Could you check a few things on this model? Use its own coordinates, in mm. A direction names the side the tool comes from. Coordinates: 2 decimals unless noted, no trailing zeros. Loops run counter-clockwise (first coordinate to the right, second up) from the corner with the lowest first, then second, coordinate; pieces in that order, holes last. Notation, with made-up numbers: (36.5, 84) - (48.5, 84) arc R28 cw to (48.5, 122) - close; hole circle Ø11 at (86, 30). An arc over 180 degrees is marked (long way). One line per item, written item: value. Start each with the question number.
(1) If we section it at B-B on y = 10.5: Write out the boundary of the cut face in (x, z).
(2) If we section it at D-D on y = 6.5: Write out the boundary of the cut face in (x, z), then the cut area to 3 significant figures.
(3) I'm going to push flat-ended pins straight in: P1, Ø10, axis at x = -13, z = -23, coming from the +Y side; P2, Ø2, axis at x = -11.5, z = -1.5, coming from the +Y side; P3, Ø0.6, axis at y = 16, z = -2, coming from the -X side. Where does each tip first touch, or does it pass through?
(4) If I drill on line 1 along X through (y, z) = (14, -10); line 2 along X through (y, z) = (1.5, -10.5); line 3 along Z through (x, y) = (-6, 6.25), over which ranges is the centre line in solid material (lowest first)? Write a range as from..to.
(5) If we mould it in two halves opening along Y, with no side actions, what happens to faces 1 (the face through (-2.54, 9, -27)), 2 (the face through (-7.96, 7.58, -1.25)), 3 (the face through (-23.45, 15.88, -51.43))? For each: pulls with the +Y half, pulls with the -Y half, needs draft (parallel to the pull), parting line crosses it, or undercut.
(6) On a 3-axis mill with a long thin cutter (end or side, diameter ignored), from which of +Z, -Z, +X, -X, +Y, -Y can I reach the whole of each face in a straight line? I mean faces 4 (the face through (-4.49, 0.64, -1.91)), 5 (the face through (-19.05, 5, -1)), 6 (the face through (-14, 10, -2.54)), 7 (the face through (-20.32, 16, -51)). Say none if no direction works.
(7) If we section it at A-A on z = -48: Count the separate pieces of the cut face and the enclosed holes in it, then the cut area to 3 significant figures.
Autodesk Inventor part; units mm, degrees
ref_plane "YZ Plane" through (0, 0, 0) normal (1, 0, 0) x (0, 1, 0)
ref_plane "XZ Plane" through (0, 0, 0) normal (0, 1, 0) x (-1, 0, 0)
ref_plane "XY Plane" through (0, 0, 0) normal (0, 0, 1) x (1, 0, 0)
sketch "Sketch1" plane through (0, 0, 0) normal (0, 1, 0) x (-1, 0, 0)
  line L0 (0, 0) -> (27.94, 0)
  line L1 (27.94, 0) -> (27.94, -53.34)
  line L2 (27.94, -53.34) -> (0, -53.34)
  line L3 (0, -53.34) -> (0, 0)
  dimension "d0" = 27.94
  dimension "d1" = 53.34
extrude "Extrusion1" add sketch "Sketch1" along normal blind 15.24
shell "Shell1" thickness 2.54 removed faces 1 at (-9.3133, 15.24, -17.78)
sketch "Sketch3" plane through (-27.94, 0, 0) normal (0, 0, 1) x (1, 0, 0)
  line L0 (21.59, 4.064) -> (8.89, 4.064)
  line L1 (8.89, 4.064) -> (8.89, 9.144)
  line L2 (8.89, 9.144) -> (21.59, 9.144)
  line L3 (21.59, 9.144) -> (21.59, 4.064)
  point P0 (27.94, 0)
  dimension "d20" = 4.064
  dimension "d21" = 12.7
  dimension "d22" = 5.08
  dimension "d23" = 6.35
extrude "Extrusion3" cut sketch "Sketch3" against normal blind 2.54
chamfer "Chamfer1" distance 3.175 angle 45 2 edges at (-19.05, 9.144, -1.27) (-6.35, 9.144, -1.27)
sketch "Sketch5" plane through (-25.4, 2.54, -2.54) normal (0, 1, 0) x (1, 0, 0)
  line L0 (0, 0) -> (5.08, 0)
  line L1 (5.08, 0) -> (5.08, 48.26)
  line L2 (5.08, 48.26) -> (0, 48.26)
  line L3 (0, 48.26) -> (0, 0)
  line L4 (0, 48.26) -> (22.86, 48.26)
  line L5 (22.86, 0) -> (17.78, 0)
  line L6 (17.78, 0) -> (17.78, 48.26)
  line L7 (17.78, 48.26) -> (22.86, 48.26)
  line L8 (22.86, 48.26) -> (22.86, 0)
  point P0 (25.4, -2.54)
  dimension "d29" = 5.08
  dimension "d30" = 5.08
extrude "Extrusion4" cut sketch "Sketch5" against normal blind 2.54
sketch "Sketch6" plane through (-27.94, 0, -53.34) normal (-1, 0, 0) x (0, 0, 1)
  point P0 (53.34, 0)
sketch "Sketch7" plane through (-27.94, 0, -53.34) normal (-1, 0, 0) x (0, 0, 1)
  line L0 (2.54, 15.24) -> (50.8, 15.24)
  line L1 (0, 0) -> (2.54, 0)
  line L2 (2.54, 0) -> (2.54, 15.24)
  line L3 (2.54, 15.24) -> (0, 15.24)
  line L4 (0, 15.24) -> (0, 0)
  point P0 (53.34, 0)
  dimension "d33" = 2.54
extrude "Extrusion5" add sketch "Sketch7" along normal blind 5.08
sketch "Sketch8" plane through (-27.94, 0, -50.8) normal (0, 0, 1) x (1, 0, 0)
  line L0 (-5.08, 15.24) -> (-2.54, 15.24)
  line L1 (-2.54, 15.24) -> (-2.54, 0)
  line L2 (-2.54, 0) -> (-5.08, 0)
  line L3 (-5.08, 0) -> (-5.08, 15.24)
  point P0 (27.94, 0)
  dimension "d36" = 2.54
extrude "Extrusion6" add sketch "Sketch8" along normal up to surface (50.8 mm away)
chamfer "Chamfer2" distance 1.27 angle 45 6 edges at (-2.54, 0, -26.67) (-5.08, 0, -2.54) (-5.08, 0, -50.8) (-22.86, 0, -2.54) (-25.4, 0, -26.67) (-22.86, 0, -50.8)
sketch "Sketch11" plane through (0, 15.24, 0) normal (0, 1, 0) x (1, 0, 0)
  line L0 (-26.67, 52.07) -> (-17.78, 52.07)
  line L1 (-20.32, 1.27) -> (-26.67, 1.27)
  line L2 (-26.67, 1.27) -> (-26.67, 52.07)
  line L3 (-25.4, 2.54) -> (-25.4, 50.8)
  line L4 (-2.54, 2.54) -> (-25.4, 2.54)
  line L5 (-25.4, 50.8) -> (-2.54, 50.8)
  line L6 (-1.27, 52.07) -> (-7.62, 52.07)
  line L7 (-7.62, 1.27) -> (-1.27, 1.27)
  line L8 (-1.27, 1.27) -> (-1.27, 52.07)
  line L9 (-2.54, 50.8) -> (-2.54, 2.54)
  line L10 (-7.62, 52.07) -> (-1.27, 52.07)
  line L11 (-1.27, 52.07) -> (-1.27, 50.8)
  line L12 (-1.27, 50.8) -> (-7.62, 50.8)
  line L13 (-7.62, 50.8) -> (-7.62, 52.07)
  line L14 (-2.54, 50.8) -> (-1.27, 50.8)
  line L15 (-1.27, 50.8) -> (-1.27, 1.27)
  line L16 (-1.27, 1.27) -> (-2.54, 1.27)
  line L17 (-2.54, 1.27) -> (-2.54, 50.8)
  line L18 (-2.54, 2.54) -> (-7.62, 2.54)
  line L19 (-7.62, 2.54) -> (-7.62, 1.27)
  line L20 (-7.62, 1.27) -> (-2.54, 1.27)
  line L21 (-2.54, 1.27) -> (-2.54, 2.54)
  line L22 (-26.67, 52.07) -> (-20.32, 52.07)
  line L23 (-20.32, 52.07) -> (-20.32, 50.8)
  line L24 (-20.32, 50.8) -> (-26.67, 50.8)
  line L25 (-26.67, 50.8) -> (-26.67, 52.07)
  line L26 (-25.4, 50.8) -> (-26.67, 50.8)
  line L27 (-26.67, 50.8) -> (-26.67, 1.27)
  line L28 (-26.67, 1.27) -> (-25.4, 1.27)
  line L29 (-25.4, 1.27) -> (-25.4, 50.8)
  line L30 (-25.4, 2.54) -> (-20.32, 2.54)
  line L31 (-20.32, 2.54) -> (-20.32, 1.27)
  line L32 (-20.32, 1.27) -> (-25.4, 1.27)
  line L33 (-25.4, 1.27) -> (-25.4, 2.54)
  point P0 (0, 0)
  dimension "d50" = 1.27
  dimension "d51" = 1.27
  dimension "d52" = 1.27
  dimension "d55" = 1.27
  dimension "d57" = 1.27
  dimension "d58" = 5.08
  dimension "d59" = 48.26
  dimension "d60" = 6.35
  dimension "d61" = 6.35
extrude "Extrusion8" add sketch "Sketch11" along normal blind 1.27 contours L0 L23 L5 L24 L2 | L24 L3 L29 L1 L2 | L13 L6 L8 L12 L5 | L29 L4 L31 L1 | L12 L8 L7 L17 L9 | L17 L7 L19 L4
chamfer "Chamfer3" distance 1.27 angle 45 6 edges at (-1.27, 16.51, -26.67) (-4.445, 16.51, -1.27) (-4.445, 16.51, -52.07) (-23.495, 16.51, -52.07) (-26.67, 16.51, -26.67) (-23.495, 16.51, -1.27)
properties part number "nano_enclosure"
Values:
1. outline: (-33.02, -53.34) - (0, -53.34) - (0, 0) - (-27.94, 0) - (-27.94, -50.8) - (-30.48, -50.8) - (-30.48, 0) - (-33.02, 0) - close; hole (-25.4, -50.8) - (-2.54, -50.8) - (-2.54, -2.54) - (-25.4, -2.54) - close
2. outline: (-33.02, -53.34) - (0, -53.34) - (0, 0) - (-6.88, 0) - (-6.88, -2.54) - (-2.54, -2.54) - (-2.54, -50.8) - (-25.4, -50.8) - (-25.4, -2.54) - (-18.52, -2.54) - (-18.52, 0) - (-27.94, 0) - (-27.94, -50.8) - (-30.48, -50.8) - (-30.48, 0) - (-33.02, 0) - close
2. area: 499 mm2
3. P1: stops at y = 2.54
3. P2: stops at y = 15.24
3. P3: stops at x = -26.21
4. line 1: x = -33.02..-30.48, -27.94..-25.4, -2.54..0
4. line 2: x = -33.02..-30.48, -27.94..-25.4, -20.32..-7.62, -2.54..0
4. line 3: z = -53.34..-50.8, -2.54..0
5. face 1: needs draft
5. face 2: undercut
5. face 3: pulls with the +Y half
6. face 4: -Y
6. face 5: +Z
6. face 6: +Y
6. face 7: +Z, -Z, +Y
7. separate pieces: 4
7. enclosed holes: 0
7. area: 148 mm2
